from build123d import *

# Parameters (mm, degrees)
SKETCH_1_W          = 52
SKETCH_1_H          = 33
SKETCH_1_W_2        = 22
SKETCH_1_H_2        = 11
EXTRUDE_1_DEPTH     = 37
SKETCH_3_W          = 13
SKETCH_3_H          = 11
CUT_EXTRUDE_1_DEPTH = 13
SKETCH_4_W          = 6
SKETCH_4_H          = 11
EXTRUDE_2_DEPTH     = 12
EXTRUDE_4_DEPTH     = 16
CUT_EXTRUDE_2_REACH = 35


with BuildPart() as part:
    # 草图1 → 凸台-拉伸1 (new body)
    with BuildSketch(Plane(origin=(0, 0, 0), x_dir=(1, 0, 0), z_dir=(0, 1, 0))):
        Rectangle(SKETCH_1_W, SKETCH_1_H)
        with Locations((-9, 0)):
            Rectangle(SKETCH_1_W_2, SKETCH_1_H_2, mode=Mode.SUBTRACT)
    extrude(amount=EXTRUDE_1_DEPTH)

    # 草图3 → 切除-拉伸1 (cut)
    with BuildSketch(Plane(origin=(0, 37, 0), x_dir=(1, 0, 0), z_dir=(0, 1, 0))):
        with Locations((8.5, 0)):
            Rectangle(SKETCH_3_W, SKETCH_3_H)
    extrude(amount=-CUT_EXTRUDE_1_DEPTH, mode=Mode.SUBTRACT)

    # 草图4 → 凸台-拉伸2 (add)
    with BuildSketch(Plane(origin=(0, 37, 0), x_dir=(1, 0, 0), z_dir=(0, 1, 0))):
        with Locations((-23, 0)):
            Rectangle(SKETCH_4_W, SKETCH_4_H)
    extrude(amount=EXTRUDE_2_DEPTH)

    # 草图6 → 凸台-拉伸4 (add)
    with BuildSketch(Plane.ZY.offset(26)):
        Polygon((5.5, 49), (16.5, 37), (5.5, 37), align=None)
    extrude(amount=-EXTRUDE_4_DEPTH)

    # 草图7 → 切除-拉伸2 (cut, up to next)
    with BuildSketch(Plane.XY.offset(16.5), mode=Mode.PRIVATE) as cut_extrude_2_sk1:
        Polygon((-20, 49), (-10, 37), (-10, 49), align=None)
    cut_extrude_2_tool1 = extrude(cut_extrude_2_sk1.sketch, amount=-CUT_EXTRUDE_2_REACH, mode=Mode.PRIVATE) & part.part
    add(cut_extrude_2_tool1.solids().sort_by_distance((-13.333333, 45, 16.5))[0], mode=Mode.SUBTRACT)


solid = part.part
The model under review builds one solid part; all positions refer to its coordinate system, in mm. A direction names the side the tool comes from. Coordinates: 2 decimals unless noted, no trailing zeros. Order: outer loops, then holes, each group sorted by start corner. A loop starts at its lowest first (then second) coordinate and runs counter-clockwise, first axis right, second up. Notation, with made-up numbers: (51.5, 10.25) -> (88.5, 10.25) arc R11 ccw to (88.5, 25.25) -> close; hole circle Ø8 at (21, 16). An arc over 180 degrees is marked (long way). Answer in a Markdown table with one row per item.
(1) Consider section C-C (z = -1.5). Write out the cut boundary in (x, y), plus the area to 3 significant figures.
Answers:
| item | result |
|---|---|
| outline | (-26, 0) -> (-20, 0) -> (-20, 49) -> (-26, 49) -> close; (2, 0) -> (26, 0) -> (26, 37) -> (15, 37) -> (15, 24) -> (2, 24) -> close |
| area | 1,010 mm² |
(2) Insertion check: pin 1 (4 mm diameter, centred on x = 14, z = 12.5, fed in from +Y); pin 2 (6.5 mm diameter, centred on x = -22, y = 44.5, fed in from -Z); pin 3 (3.5 mm diameter, centred on x = 9, z = 0, fed in from +Y). Each pin has a flat end and moves straight along its axis. Give the tip position at first contact, or say it passes through.
Answers:
| item | result |
|---|---|
| pin 1 | y = 37 |
| pin 2 | z = -5.5 |
| pin 3 | y = 24 |
(3) Consider section A-A (y = 35.5). Write out the cut boundary in (x, z), plus the area to 3 significant figures.
Answers:
| item | result |
|---|---|
| outline | (-26, -16.5) -> (26, -16.5) -> (26, 16.5) -> (-26, 16.5) -> close; hole (-20, -5.5) -> (15, -5.5) -> (15, 5.5) -> (-20, 5.5) -> close |
| area | 1,330 mm² |
(4) Machinability: for faces 1 (the flat face through (2, 12, 0)), 2 (the flat face through (0, 18, 16.5)), 3 (the flat face through (-23, 43, -5.5)), 4 (the flat face through (15, 31, 0)), 5 (the flat face through (5, 0, 0)), which of the approach directions +Z, -Z, +X, -X, +Y, -Y give a long, thin tool a straight path to every point of the face, cutting with its end or side? Answer none if there is none.
Answers:
| item | result |
|---|---|
| face 1 | +Y, -Y |
| face 2 | +Z, +X, -X, +Y, -Y |
| face 3 | -Z, +X, -X, +Y |
| face 4 | +Y |
| face 5 | +Z, -Z, +X, -X, -Y |
(5) Wall thickness on line 1 along Z through (x, y) = (0, 21); line 2 along X through (y, z) = (3, 1); line 3 along Y through (x, z) = (16.5, 13.5): over which ranges is each line inside the solid? List them lowest first.
Answers:
| item | result |
|---|---|
| line 1 | -16.5 to -5.5, 5.5 to 16.5 |
| line 2 | -26 to -20, 2 to 26 |
| line 3 | 0 to 37 |
(6) Consider section D-D (x = 10.5). Write out the cut boundary in (y, z), plus the area to 3 significant figures.
Answers:
| item | result |
|---|---|
| outline | (0, -16.5) -> (37, -16.5) -> (37, -5.5) -> (24, -5.5) -> (24, 5.5) -> (37, 5.5) -> (37, 16.5) -> (0, 16.5) -> close |
| area | 1,080 mm² |
(7) The part is to be moulded in two halves that separate along X. For faces 6 (the flat face through (-12.85, 40.42, 8.63)), 7 (the flat face through (-7, 24, 5.5)), 8 (the flat face through (5, 37, -8)), say which applies: +X half, -X half, draft (parallel to the pull), parting line (faces both ways), or undercut.
Answers:
| item | result |
|---|---|
| face 6 | +X half |
| face 7 | undercut |
| face 8 | draft |
(8) Consider section B-B (x = -8). Write out the cut boundary in (y, z), plus the area to 3 significant figures.
Answers:
| item | result |
|---|---|
| outline | (0, -16.5) -> (37, -16.5) -> (37, -5.5) -> (0, -5.5) -> close; (0, 5.5) -> (37, 5.5) -> (37, 16.5) -> (0, 16.5) -> close |
| area | 814 mm² |
